Autodesk Inventor part; units mm, degrees
ref_plane "YZ Plane" through (0, 0, 0) normal (1, 0, 0) x (0, 1, 0)
ref_plane "XZ Plane" through (0, 0, 0) normal (0, 1, 0) x (-1, 0, 0)
ref_plane "XY Plane" through (0, 0, 0) normal (0, 0, 1) x (1, 0, 0)
sketch "Szkic1" plane through (0, 0, 0) normal (1, 0, 0) x (0, 1, 0)
  line L0 (10, 0) -> (10, 0)
  line L1 (20, 10) -> (20, 210)
  line L2 (10, 220) -> (10, 220)
  line L3 (0, 210) -> (0, 10)
  arc A0 (20, 210) -> (10, 220) centre (10, 210) ccw
  arc A1 (10, 220) -> (0, 210) centre (10, 210) ccw
  arc A2 (10, 0) -> (20, 10) centre (10, 10) ccw
  arc A3 (0, 10) -> (10, 0) centre (10, 10) ccw
  circle A4 centre (10, 210) radius 1.6
  circle A5 centre (10, 70) radius 1.6
  circle A6 centre (10, 10) radius 1.6
  point P0 (0, 0)
  point P1 (20, 220)
  point P2 (0, 220)
  dimension "d0" = 20
  dimension "d1" = 10
  dimension "d2" = 200
  dimension "d3" = 60
  dimension "d4" = 3.2
  dimension "d5" = 3.2
  dimension "d6" = 3.2
extrude "Wyciągnięcie proste1" add sketch "Szkic1" along normal blind 3
properties part number "segment2"
Geometry check sheet. Reference: the model listing, model coordinates, mm. Coordinates: 2 decimals unless noted, no trailing zeros. Order: outer loops, then holes, each group sorted by start corner. A loop starts at its lowest first (then second) coordinate and runs counter-clockwise, first axis right, second up. Notation, with made-up numbers: (61, 0) - (90, 0) arc R29 cw to (90, 37) - close; hole circle Ø4 at (5, 25.5). An arc over 180 degrees is marked (long way). Answer in a Markdown table with one row per item. Add a question column.
1) Gauge pin test, flat end, axial feed: P1, Ø1, axis at x = 1.5, y = 3, coming from the +Z side. Record the tip position at first contact, or that the pin passes through.
2) Cross-section at A-A, the plane x = 2. Record the cut outline in (y, z), then the cut area to 3 significant figures.
3) Material ranges on line 1 along Z through (x, y) = (1.6, 10); line 2 along Y through (x, z) = (1.45, 70); line 3 along Z through (x, y) = (2.3, 9.25), recorded low to high. Write a range as [from, to].
Check result:
| question | item | result |
|---|---|---|
| 1 | P1 | stops at z = 217.6 |
| 2 | outline | (0, 10) arc R10 ccw to (20, 10) - (20, 210) arc R10 ccw to (0, 210) - close; hole circle Ø3.2 at (10, 10); hole circle Ø3.2 at (10, 70); hole circle Ø3.2 at (10, 210) |
| 2 | area | 4,290 mm² |
| 3 | line 1 | z = [0, 8.4], [11.6, 68.4], [71.6, 208.4], [211.6, 220] |
| 3 | line 2 | y = [0, 8.4], [11.6, 20] |
| 3 | line 3 | z = [0.03, 8.59], [11.41, 68.59], [71.41, 208.59], [211.41, 219.97] |
